from build123d import *

# Parameters (mm, degrees)
ESQUISSE1_R        = 25
BOSS_EXTRU_1_DEPTH = 5


with BuildPart() as part:
    # Esquisse1 → Boss.-Extru.1 (new body)
    with BuildSketch(Plane.XY):
        Circle(ESQUISSE1_R)
        with BuildLine():
            Line((14.953030626, -4.277181575), (16.501758042, -4.982426557))
            ThreePointArc((16.501758042, -4.982426557), (16.651785463, -5.134087079), (16.663083329, -5.347116418))
            ThreePointArc((16.663083329, -5.347116418), (15.924531384, -7.256672806), (14.968008895, -9.066901881))
            ThreePointArc((14.968008895, -9.066901881), (14.799864591, -9.198133844), (14.587009397, -9.184458985))
            Line((14.587009397, -9.184458985), (13.038282108, -8.478683252))
            ThreePointArc((13.038282108, -8.478683252), (12.832759155, -8.462847948), (12.665533258, -8.583371557))
            ThreePointArc((12.665533258, -8.583371557), (-13.922503409, 6.344596033), (14.787409001, -3.927153556))
            ThreePointArc((14.787409001, -3.927153556), (14.806182583, -4.132467854), (14.953030626, -4.277181575))
        make_face(mode=Mode.SUBTRACT)
    extrude(amount=BOSS_EXTRU_1_DEPTH)


solid = part.part
Read the model definition and answer for the solid it produces. Units are mm, in the model's axes. A direction names the side the tool comes from. Give positions to 0.01 mm unless a question says otherwise; leave off trailing zeros. Loops run counter-clockwise (first coordinate to the right, second up) from the corner with the lowest first, then second, coordinate; pieces in that order, holes last. Notation, with made-up numbers: (87.25, 15.5) -> (109.25, 15.5) arc R33 cw to (109.25, 44.5) -> close; hole circle Ø3 at (26, 17.25). An arc over 180 degrees is marked (long way). Answer as CSV lines item,"result".
Item 1: Consider line 1 (Y direction, x = 0, z = 1.8); line 2 (X direction, y = -2, z = 4.8); line 3 (X direction, y = 1.5, z = 2.8). Determine where each line is inside the solid, lowest interval first. Write a range as [from, to].
Returned:
line 1,"y = [-25, -15.3], [15.3, 25]"
line 2,"x = [-24.92, -15.17], [15.17, 24.92]"
line 3,"x = [-24.95, -15.23], [15.23, 24.95]"
Item 2: Find section D-D on y = 20.5. Give the vertices of the cut face in (x, z), plus the area to 3 significant figures.
Returned:
outline,"(-14.31, 0) -> (14.31, 0) -> (14.31, 5) -> (-14.31, 5) -> close"
area,"143 mm²"
Item 3: Determine the mould class of faces 1 (the face through (13.823, -8.837, 2.465)), 2 (the face through (23.846, 7.509, 2.465)), 3 (the face through (-11, -11, 0)) for opening direction X: +X half, -X half, draft (parallel to the pull), parting line (faces both ways), or undercut.
Returned:
face 1,"undercut"
face 2,"parting line"
face 3,"draft"
Item 4: Each of these flat-tipped pins is pushed along its axis until it touches: pin 1 (1.5 mm diameter, centred on x = 2.5, y = 12.5, fed in from -Z); pin 2 (1.5 mm diameter, centred on y = 2.5, z = 1, fed in from -X); pin 3 (1 mm diameter, centred on y = 15.5, z = 3, fed in from +X); pin 4 (1 mm diameter, centred on y = 5, z = 2.5, fed in from -X). Where does it stop, or does it pass through?
Returned:
pin 1,"passes through"
pin 2,"stops at x = -24.94"
pin 3,"stops at x = 20"
pin 4,"stops at x = -24.59"
Item 5: Find section C-C on z = 3.15. Give the vertices of the cut face in (x, y).
Returned:
outline,"circle Ø50 at (0, 0); hole (12.67, -8.58) arc R0.3 cw to (13.04, -8.48) -> (14.59, -9.18) arc R0.3 ccw to (14.97, -9.07) arc R17.5 ccw to (16.66, -5.35) arc R0.3 ccw to (16.5, -4.98) -> (14.95, -4.28) arc R0.3 cw to (14.79, -3.93) arc R15.3 ccw (long way) to start"
Item 6: Find section A-A on y = 0. Give the vertices of the cut face in (x, z).
Returned:
outline,"(-25, 0) -> (-15.3, 0) -> (-15.3, 5) -> (-25, 5) -> close; (15.3, 0) -> (25, 0) -> (25, 5) -> (15.3, 5) -> close"
Item 7: For faces 4 (the face through (-11, -11, 5)), 5 (the face through (15.936, -7.231, 2.465)), determine the directions among +Z, -Z, +X, -X, +Y, -Y from which every point of the face is accessible in a straight line to the end or side of a thin tool.
Returned:
face 4,"+Z, +X, -X, +Y, -Y"
face 5,"+Z, -Z"
